from build123d import *

# Parameters (mm, degrees)
SKETCH1_W           = 110
SKETCH1_H           = 130
BOSS_EXTRUDE1_DEPTH = 200
SHELL1_T            = -5
SKETCH2_W           = 110
SKETCH2_H           = 1.7
BOSS_EXTRUDE2_DEPTH = 200
SKETCH5_W           = 110
SKETCH5_H           = 3
BOSS_EXTRUDE3_DEPTH = 200


with BuildPart() as part:
    # Sketch1 → Boss-Extrude1 (new body)
    with BuildSketch(Plane.XY):
        Rectangle(SKETCH1_W, SKETCH1_H)
    extrude(amount=BOSS_EXTRUDE1_DEPTH)

    # Shell1
    shell1_openings = [part.faces().sort_by_distance(p)[0] for p in [
        (0, 0, 200),
    ]]
    offset(amount=SHELL1_T, openings=shell1_openings, kind=Kind.INTERSECTION)

    # Sketch2 → Boss-Extrude2 (add)
    with BuildSketch(Plane(origin=(0, 0, 0), x_dir=(-1, 0, 0), z_dir=(0, 0, -1))):
        with Locations((0, 2.15)):
            Rectangle(SKETCH2_W, SKETCH2_H)
    extrude(amount=-BOSS_EXTRUDE2_DEPTH)

    # Sketch5 → Boss-Extrude3 (add)
    with BuildSketch(Plane(origin=(0, 0, 0), x_dir=(-1, 0, 0), z_dir=(0, 0, -1))):
        with Locations((0, 41.5)):
            Rectangle(SKETCH5_W, SKETCH5_H)
    extrude(amount=-BOSS_EXTRUDE3_DEPTH)


solid = part.part
Input: part model. Units: mm. Frame: model coordinates. A direction names the side the tool comes from. Give positions to 0.01 mm unless a question says otherwise; leave off trailing zeros. Order: outer loops, then holes, each group sorted by start corner. A loop starts at its lowest first (then second) coordinate and runs counter-clockwise, first axis right, second up.
Q1. Contact query for a flat-ended pin moving along its axis: pin 1 Ø5 at (x, y) = (-25, 53.5) entering from +Z. Output: stop coordinate, or through.
Checked values:
pin 1: stops at z = 5
Q2. Section A-A on z = 68.5. Output: boundary loops of the cut face in (x, y).
Checked values:
outline: (-55, -65) - (55, -65) - (55, 65) - (-55, 65) - close; hole (-50, -60) - (50, -60) - (50, 1.3) - (-50, 1.3) - close; hole (-50, 3) - (50, 3) - (50, 40) - (-50, 40) - close; hole (-50, 43) - (50, 43) - (50, 60) - (-50, 60) - close
Q3. Draft query along X for faces 1 (the flat face through (1, 1, 0)), 2 (the flat face through (-1, 60, 101)), 3 (the flat face through (55, -1, 99)), 4 (the flat face through (1, 3, 101)). Return one class per face: +X half, -X half, draft (parallel to the pull), parting line (faces both ways), or undercut.
Checked values:
face 1: draft
face 2: undercut
face 3: +X half
face 4: undercut
Q4. Set-up query: faces 5 (the flat face through (-1, -65, 99)), 6 (the flat face through (-1, 22, 5)). Return all of +Z, -Z, +X, -X, +Y, -Y with unobstructed straight access to the full face (end or side cutting, diameter ignored); none if empty.
Checked values:
face 5: +Z, -Z, +X, -X, -Y
face 6: +Z
Q5. Ray query, probe 1 along Y at (x, z) = (29.5, 141); probe 2 along X at (y, z) = (25, 81.5); probe 3 along Z at (x, y) = (48.5, -22). Return the intervals inside material, ascending.
Checked values:
probe 1: y = -65 to -60, 1.3 to 3, 40 to 43, 60 to 65
probe 2: x = -55 to -50, 50 to 55
probe 3: z = 0 to 5
Q6. Section B-B on y = 54. Output: boundary loops of the cut face in (x, z).
Checked values:
outline: (-55, 0) - (55, 0) - (55, 200) - (50, 200) - (50, 5) - (-50, 5) - (-50, 200) - (-55, 200) - close
Q7. Section C-C on x = -13.5. Output: boundary loops of the cut face in (y, z).
Checked values:
outline: (-65, 0) - (65, 0) - (65, 200) - (60, 200) - (60, 5) - (43, 5) - (43, 200) - (40, 200) - (40, 5) - (3, 5) - (3, 200) - (1.3, 200) - (1.3, 5) - (-60, 5) - (-60, 200) - (-65, 200) - close
